Part model, mm, in its own coordinate system. A direction names the side the tool comes from. Round coordinates to 2 decimals unless told otherwise and drop trailing zeros. Loops run counter-clockwise (first coordinate to the right, second up) from the corner with the lowest first, then second, coordinate; pieces in that order, holes last. Notation, with made-up numbers: M 77.5,45.25 L 102.5,45.25 A33 cw 102.5,73.25 Z; hole C 59,23 d8. An arc over 180 degrees is marked long. Write each question's results on one line, items separated by ' | '.
from build123d import *

# Parameters (mm, degrees)
EXTRUDE_1_DEPTH     = 8
EXTRUDE_2_DEPTH     = 20
HOLE_WIZARD_M5_1_D  = 5.3
FILLET_1_R          = 7.5
FILLET_2_DEPTH      = 8
SKETCH_5_W          = 3.1999999999999886
SKETCH_5_H          = 8.2
FILLET_3_R          = 1.5
FILLET_4_R          = 1.5
CUT_EXTRUDE_1_DEPTH = 5


with BuildPart() as part:
    # 草图1 → 凸台-拉伸1 (new body)
    with BuildSketch(Plane(origin=(0, 0, 0), x_dir=(1, 0, 0), z_dir=(0, 1, 0))):
        with BuildLine():
            Line((2.098e-14, -189), (1.932e-14, -174.00000000000003))
            ThreePointArc((2.28618e-12, -174.00000000000003), (-15.165099238093463, -173.33787746796366), (-30.214782914050144, -171.35654902412347))
            Line((-30.214782914045937, -171.35654902412418), (-32.8195055790499, -186.12866531930732))
            ThreePointArc((-32.81950557905, -186.12866531930732), (-16.472435379307413, -188.28079793933995), (-3.472e-14, -189.00000000000003))
        make_face()
    extrude(amount=EXTRUDE_1_DEPTH)

    # 草图4 → 凸台-拉伸2 (add)
    with BuildSketch(Plane(origin=(0, 8, 0), x_dir=(1, 0, 0), z_dir=(0, 1, 0))):
        with BuildLine():
            Line((2.082e-14, -189), (1.916e-14, -174))
            ThreePointArc((-3.196e-14, -174.00000000000003), (-1.5184171767173116, -173.99337461316583), (-3.0367187200877925, -173.9734989572121))
            Line((-3.036718720087315, -173.97349895721206), (-3.298504816646567, -188.97121438455795))
            ThreePointArc((-3.2985048166465822, -188.971214384558), (-1.6493152091926062, -188.99280345912842), (-3.472e-14, -189.00000000000006))
        make_face()
    extrude(amount=EXTRUDE_2_DEPTH)

    # M5 间隙孔1 (through all)
    with Locations(Plane(origin=(0, 8, 0), x_dir=(1, 0, 0), z_dir=(0, 1, 0))):
        with Locations((-23.608051681, -179.958078162), (-11.163314825, -181.156370029)):
            Hole(HOLE_WIZARD_M5_1_D / 2)

    # 圆角1
    # the kernel refuses this fillet: 7.5 mm, written as the material it takes off along each edge
    with BuildSketch(Plane(origin=(1.47232e-12, 28, -1.0760459e-10), x_dir=(0.10755019962978496, 0, 0.9941996552803635), z_dir=(0.9941996552803635, 0, -0.10755019962978496))) as fillet_1_piece_1:
        with BuildLine():
            CenterArc((174.00000000010766 + FILLET_1_R, FILLET_1_R), FILLET_1_R, 180, 89.99999999999977)
            Line((174.00000000010766 + FILLET_1_R, 0), (174.00000000010766, 0))
            Line((174.00000000010766, 0), (174.00000000010766, FILLET_1_R))
        make_face()
    revolve(axis=Axis((1.47232e-12, 28, -1.0760459e-10), (0, -1, 0)), revolution_arc=13.348228955549553, mode=Mode.SUBTRACT)
    with BuildSketch(Plane(origin=(2.05469e-12, 28, -2.9481839e-10), x_dir=(-0.11639521392683701, 0, 0.9932029773288671), z_dir=(-0.9932029773288671, 0, -0.11639521392683701))) as fillet_1_piece_2:
        with BuildLine():
            CenterArc((189.0000000002949 - FILLET_1_R, -FILLET_1_R), FILLET_1_R, 0, 89.99999999999957)
            Line((189.0000000002949 - FILLET_1_R, 0), (189.0000000002949, 0))
            Line((189.0000000002949, 0), (189.00000000029488, -FILLET_1_R))
        make_face()
    revolve(axis=Axis((2.05469e-12, 28, -2.9481839e-10), (0, 1, 0)), revolution_arc=12.368210784462358, mode=Mode.SUBTRACT)

    # 圆角2: read off the stored shape, not the designer's step
    # 圆角2 outline → 圆角2 (cut)
    with BuildSketch(Plane(origin=(0, 0, 0), x_dir=(1, 0, 0), z_dir=(0, 1, 0))):
        with BuildLine():
            ThreePointArc((-32.819505579, -186.128665319), (-28.966041771, -186.767150281), (-25.100206236, -187.325864863))
            add(Edge.make_bspline(
                [(-25.100206236, -187.325864863), (-27.006863278382305, -187.07038767754574), (-29.132080374521447, -186.17341393049847), (-31.048536919413714, -184.35464406978926), (-32.02623112721157, -181.62978297542463), (-31.490224503, -178.589937725)],
                knots=[0, 0, 0, 0, 0, 0, 0.5103349834155644, 0.5103349834155644, 0.5103349834155644, 0.5103349834155644, 0.5103349834155644, 0.5103349834155644], degree=5, weights=[1, 0.7958660065557144, 0.6438203721908997, 0.5438630969055563, 0.4959941806996843, 0.5002136235732837]))
            Line((-31.490224503, -178.589937725), (-32.819505579, -186.128665319))
        make_face()
        with BuildLine():
            Line((-30.214782914, -171.356549024), (-31.490224503, -178.589937725))
            add(Edge.make_bspline(
                [(-31.490224503, -178.589937725), (-30.984360135627078, -175.72103774319677), (-29.29551148466263, -173.58668082656104), (-27.075163325391554, -172.48015181385665), (-24.918748626576246, -172.21612345785414), (-23.108126376, -172.458732732)],
                knots=[0.5103349834155644, 0.5103349834155644, 0.5103349834155644, 0.5103349834155644, 0.5103349834155644, 0.5103349834155644, 1, 1, 1, 1, 1, 1], degree=5, weights=[0.5002136235732837, 0.5042621674352976, 0.5562650770089762, 0.6562223522943196, 0.8041339932913276, 1]))
            ThreePointArc((-23.108126376, -172.458732732), (-26.667149567, -171.944360576), (-30.214782914, -171.356549024))
        make_face()
    extrude(amount=FILLET_2_DEPTH, mode=Mode.SUBTRACT)

    # 草图5 → 切除-旋转1 (revolve, cut)
    with BuildSketch(Plane(origin=(0, 0, 0), x_dir=(-0.01745240643728342, 0, 0.9998476951563913), z_dir=(-0.9998476951563913, 0, -0.01745240643728342))):
        with Locations((181.5, 20.99999999999998)):
            Rectangle(SKETCH_5_W, SKETCH_5_H)
    revolve(axis=Axis((0, 55.00000000000001, 0), (0, -1, 0)), mode=Mode.SUBTRACT)

    # 圆角3
    fillet_3_edges = [part.edges().sort_by_distance(p)[0] for p in [
        (-1.5978286497523058, 25.09999999999998, 183.09302811304977),
        (-1.5978286497523058, 16.899999999999984, 183.09302811304977),
        (-1.5699037361575081, 16.899999999999984, 179.89314995924443),
        (-1.5699037361575081, 25.09999999999998, 179.89314995924443),
    ]]
    fillet(fillet_3_edges, radius=FILLET_3_R)

    # 圆角4
    fillet_4_edges = [part.edges().sort_by_distance(p)[0] for p in [
        (-8.49e-15, 10.25, 189.00000000000003),
        (-3.2985048166465747, 14.25, 188.97121438455798),
        (-3.0367187200875536, 14.25, 173.9734989572121),
        (7.2842e-13, 10.25, 174.00000000000003),
        (-1.5838661929530051, 28, 181.4930890361471),
        (-1.5838661929530051, 28, 181.4930890361471),
    ]]
    fillet(fillet_4_edges, radius=FILLET_4_R)

    # 草图6 → 切除-拉伸1 (cut)
    with BuildSketch(Plane.XZ):
        Polygon((-23.608051681342282, 175.2815409817045), (-19.55805168134228, 177.6198095719225), (-19.55805168134228, 182.29634675235855), (-23.608051681342257, 184.6346153425765), (-27.658051681342297, 182.29634675235852), (-27.658051681342297, 177.6198095719225), align=None)
        Polygon((-11.163314825368898, 176.479832848635), (-7.113314825368922, 178.81810143885298), (-7.1133148253689225, 183.49463861928896), (-11.163314825368879, 185.83290720950694), (-15.213314825368883, 183.49463861928893), (-15.213314825368883, 178.81810143885298), align=None)
    extrude(amount=-CUT_EXTRUDE_1_DEPTH, mode=Mode.SUBTRACT)


solid = part.part
Item 1: Drop flat-ended pins along their axis: P1, Ø2, axis at x = -11.5, z = 175, coming from the +Y side; P2, Ø3, axis at x = -3.5, z = 184, coming from the +Y side; P3, Ø4, axis at y = 24, z = 180, coming from the -X side. Give the stop position or say it passes through.
Filled sheet:
P1: y = 8 | P2: y = 27.7 | P3: x = -3.17
Item 2: Wall check: L1, parallel to Y at x = -20, z = 175; L2, parallel to X at y = 10, z = 187.5; L3, parallel to Z at x = -21, y = 3. Give the ranges that are in metal, low to high.
Filled sheet:
L1: 0 to 8 | L2: -3.27 to 0 | L3: 172.73 to 176.79, 183.13 to 187.83
Item 3: Which spindle directions (+Z, -Z, +X, -X, +Y, -Y) get a long thin tool onto all of the face, cutting with end or side? Do faces 5 (the flat face through (-21.555, 2.465, 183.449)), 6 (the flat face through (0, 13, 182)). Say none if no direction does.
Filled sheet:
face 5: -Y | face 6: +Z, -Z, +X, +Y, -Y
Item 4: Band-saw the part on B-B on y = 17.75. Give the cut face in (x, z), and give its area (3 significant figures).
Filled sheet:
outline: M -3.27,187.47 L -3.19,182.92 A182.95 cw 0,182.95 L 0,187.49 A1.5 ccw -1.51,188.99 A189 ccw -1.79,188.99 A1.5 ccw Z; M -3.14,180.02 L -3.06,175.47 A1.5 ccw -1.55,173.99 A174 cw -1.49,173.99 A1.5 ccw 0,175.49 L 0,180.05 A180.05 ccw Z | area: 36.4 mm^2
Item 5: Two-plate mould, pull along Y, no slides. Class faces 1 (the flat face through (-26.4, 5, 179)), 2 (the flat face through (-25.605, 2.465, 183.482)), 3 (the cylindrical face through (-1.575, 21.036, 183.093)), 4 (the cylindrical face through (-1.548, 21.036, 179.893)): +Y half, -Y half, draft (parallel to the pull), parting line (faces both ways), or undercut.
Filled sheet:
face 1: -Y half | face 2: draft | face 3: undercut | face 4: undercut
Item 6: Band-saw the part on A-A on y = 14.5. Give the cut face in (x, z), and give its area (3 significant figures).
Filled sheet:
outline: M -3.27,187.47 L -3.06,175.47 A1.5 ccw -1.55,173.99 A174 cw -1.49,173.99 A1.5 ccw 0,175.49 L 0,187.49 A1.5 ccw -1.51,188.99 A189 ccw -1.79,188.99 A1.5 ccw Z | area: 45.6 mm^2
Item 7: Band-saw the part on C-C on x = -18. Give the cut face in (y, z).
Filled sheet:
outline: M 0,173.07 L 8,173.07 L 8,188.14 L 0,188.14 Z
